Geometry: see drawing. Coordinates: mm, zero at the bounding-box minimum. Coordinates: 2 decimals unless noted, no trailing zeros. Write each loop counter-clockwise with the first axis right and the second up, starting at its lowest first coordinate (ties: lowest second). Pieces come first, ordered by that corner, then holes. Notation, with made-up numbers: (26.25, 67.25) - (68.25, 67.25) arc R26 ccw to (68.25, 92.25) - close; hole circle Ø2 at (-39.75, -22.75). An arc over 180 degrees is marked (long way). One line per question, with ' | ' between items. Start each with the question number.
1) Line query: line 1 (Z direction, x = 50.8, y = 43); line 2 (Y direction, x = 51.5, z = 63.5); line 3 (X direction, y = 71, z = 52.5). Output: solid intervals per line, ascending.
2) First-contact query: P1, Ø5, axis at x = 48, y = 66, coming from the +Z side; P2, Ø1.5, axis at x = 45, y = 80.5, coming from the -Z side; P3, Ø4, axis at y = 55.5, z = 89, coming from the +X side. Flat tips, straight axial feed; report the tip coordinate or a pass-through.
3) Draft query along Z for the marked faces 1, 2 and 3. Return one class per face: released by +Z, released by -Z, zero draft, split by the parting line, or undercut.
4) Section query B-B on y = 21.5. Return loops of the section in (x, z).
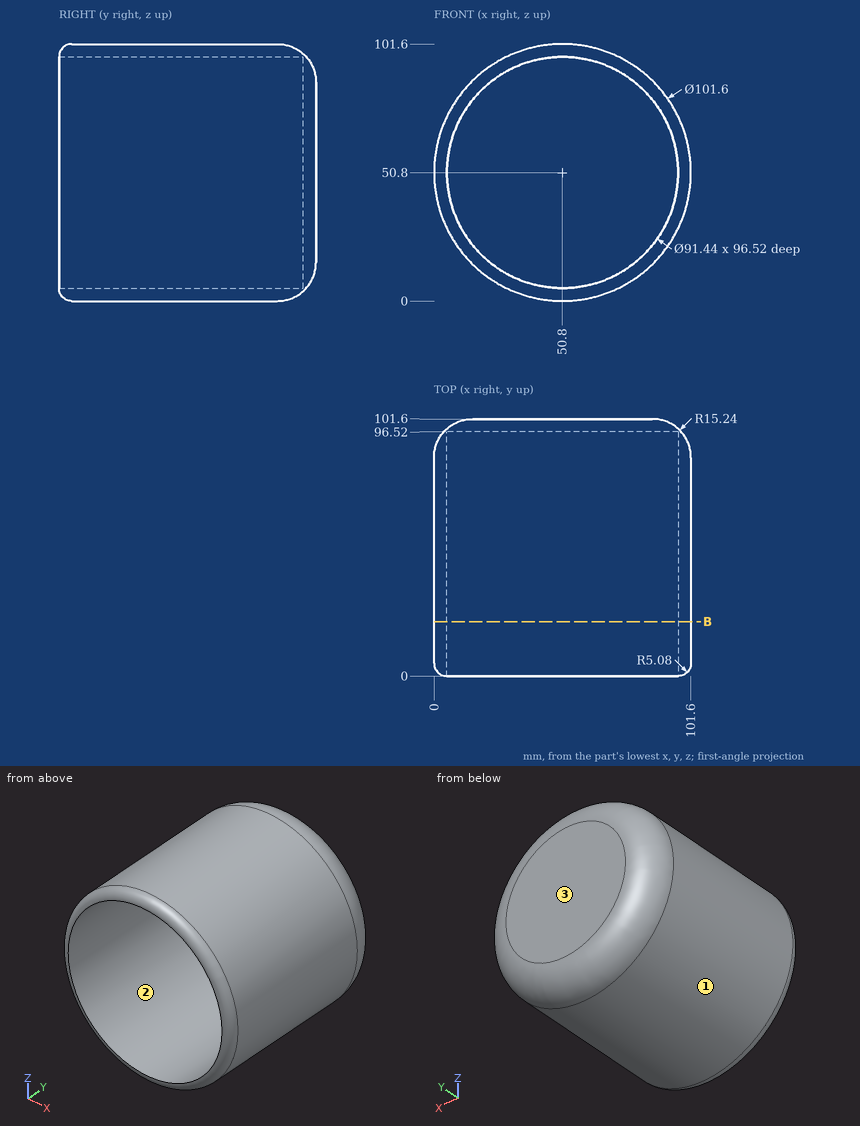
Answer key:
1) line 1: 0 to 5.08, 96.52 to 101.6 | line 2: 96.52 to 101.6 | line 3: 0.03 to 5.11, 96.49 to 101.57
2) P1: z = 101.6 | P2: z = 0.25 | P3: x = 86.44
3) face 1: split by the parting line | face 2: undercut | face 3: zero draft
4) outline: circle Ø101.6 at (50.8, 50.8); hole circle Ø91.44 at (50.8, 50.8)
